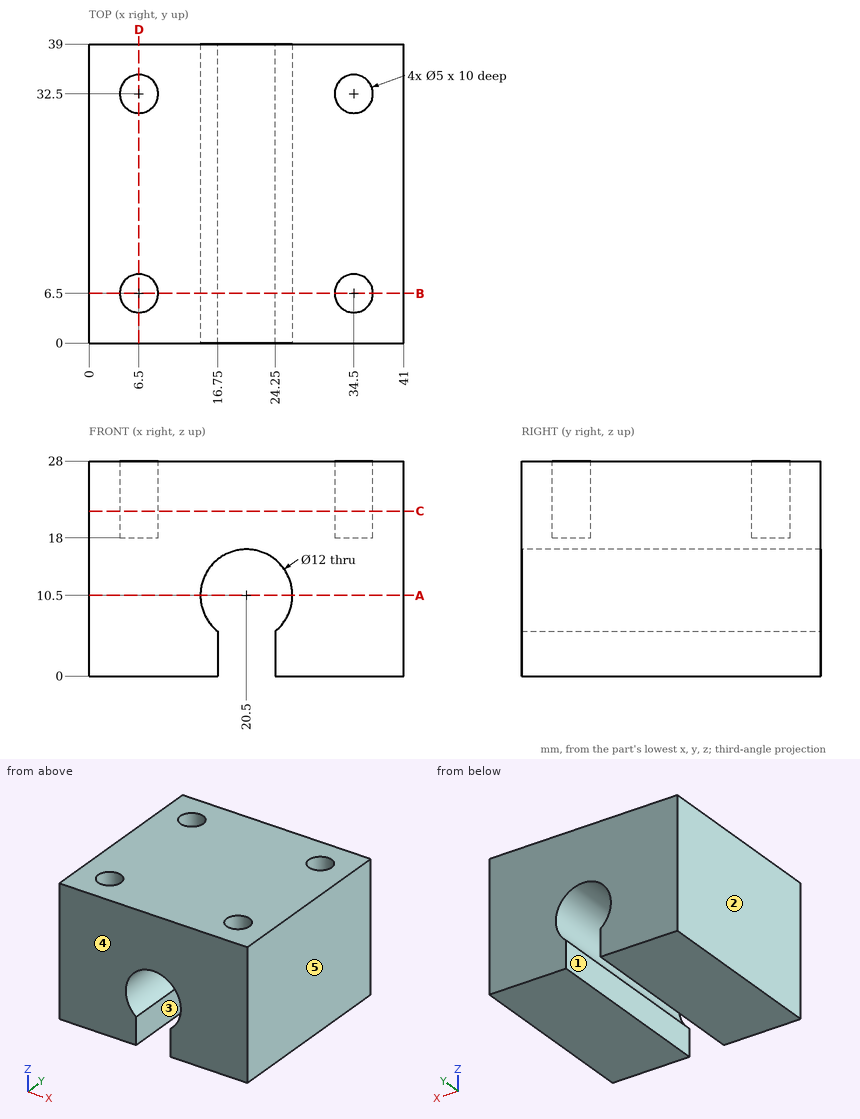
Study the drawing (mm; zero at the part's minimum x, y, z) and answer. A direction names the side the tool comes from. Round coordinates to 2 decimals unless told otherwise and drop trailing zeros. Write each loop counter-clockwise with the first axis right and the second up, starting at its lowest first coordinate (ties: lowest second). Pieces come first, ordered by that corner, then holes.
1) A cutting plane is placed at D-D on x = 6.5. Determine the outline of the cut face in (y, z), and give its area (3 significant figures).
2) A cutting plane is placed at B-B on y = 6.5. Determine the outline of the cut face in (x, z).
3) A cutting plane is placed at A-A on z = 10.5. Determine the outline of the cut face in (x, y), and give its area (3 significant figures).
4) A cutting plane is placed at C-C on z = 21.5. Determine the outline of the cut face in (x, y).
5) Determine the mould class of the marked faces 3, 4 and 5 for opening direction X: pulls with the +X half, pulls with the -X half, needs draft (parallel to the pull), parting line crosses it, or undercut.
6) Which of the six approach directions +Z, -Z, +X, -X, +Y, -Y give full straight-line access (tool end or side, diameter ignored) to the marked faces 1 and 2?
7) Flat-ended cylindrical pins translate along their axes: P1, Ø3, axis at x = 6.5, y = 32.5, coming from the +Z side; P2, Ø11, axis at x = 20.5, z = 10.5, coming from the -Y side. Find the tip coordinate at first contact, or state that the pin passes through.
8) Consider probe 1 along Y at (x, z) = (34.5, 20); probe 2 along X at (y, z) = (6.5, 23.25); probe 3 along X at (y, z) = (10, 10.5). Determine where each line is inside the solid, lowest interval first.
Entries:
1. outline: (0, 0) - (39, 0) - (39, 28) - (35, 28) - (35, 18) - (30, 18) - (30, 28) - (9, 28) - (9, 18) - (4, 18) - (4, 28) - (0, 28) - close
1. area: 992 mm2
2. outline: (0, 0) - (16.75, 0) - (16.75, 5.82) arc R6 cw (long way) to (24.25, 5.82) - (24.25, 0) - (41, 0) - (41, 28) - (37, 28) - (37, 18) - (32, 18) - (32, 28) - (9, 28) - (9, 18) - (4, 18) - (4, 28) - (0, 28) - close
3. outline: (0, 0) - (14.5, 0) - (14.5, 39) - (0, 39) - close; (26.5, 0) - (41, 0) - (41, 39) - (26.5, 39) - close
3. area: 1,130 mm2
4. outline: (0, 0) - (41, 0) - (41, 39) - (0, 39) - close; hole circle Ø5 at (6.5, 6.5); hole circle Ø5 at (6.5, 32.5); hole circle Ø5 at (34.5, 6.5); hole circle Ø5 at (34.5, 32.5)
5. face 3: undercut
5. face 4: needs draft
5. face 5: pulls with the +X half
6. face 1: -Z, +Y, -Y
6. face 2: +Z, -Z, -X, +Y, -Y
7. P1: stops at z = 18
7. P2: passes through
8. probe 1: y = 0 to 4, 9 to 30, 35 to 39
8. probe 2: x = 0 to 4, 9 to 32, 37 to 41
8. probe 3: x = 0 to 14.5, 26.5 to 41
